from build123d import *

# Parameters (mm, degrees)
F0_W     = 15.8
F0_H     = 31.8
F0_R     = 2.4
F1_DEPTH = 9.6
F2_DEPTH = 11.4
F3_T     = -1.2
F5_W     = 0.6
F5_H     = 0.6
F6_DEPTH = 8.4
F4_R     = 3.25
F4_R_2   = 2.4
F7_DEPTH = 8.4
F8_START = 1.5
F8_DEPTH = 6.9


with BuildPart() as f1:
    # F0 (on Top) → F1 (new body)
    with BuildSketch(Plane.XY):
        Rectangle(F0_W, F0_H)
        with Locations((-4, -12)):
            Circle(F0_R, mode=Mode.SUBTRACT)
        with Locations((-4, -4)):
            Circle(F0_R, mode=Mode.SUBTRACT)
        with Locations((4, -12)):
            Circle(F0_R, mode=Mode.SUBTRACT)
        with Locations((4, -4)):
            Circle(F0_R, mode=Mode.SUBTRACT)
        with Locations((-4, 4)):
            Circle(F0_R, mode=Mode.SUBTRACT)
        with Locations((-4, 12)):
            Circle(F0_R, mode=Mode.SUBTRACT)
        with Locations((4, 4)):
            Circle(F0_R, mode=Mode.SUBTRACT)
        with Locations((4, 12)):
            Circle(F0_R, mode=Mode.SUBTRACT)
        with Locations((4, 4)):
            Circle(F0_R)
        with Locations((4, 12)):
            Circle(F0_R)
        with Locations((4, -4)):
            Circle(F0_R)
        with Locations((4, -12)):
            Circle(F0_R)
        with Locations((-4, -12)):
            Circle(F0_R)
        with Locations((-4, -4)):
            Circle(F0_R)
        with Locations((-4, 4)):
            Circle(F0_R)
        with Locations((-4, 12)):
            Circle(F0_R)
    extrude(amount=F1_DEPTH)

    # F0 (on Top) → F2 (join)
    with BuildSketch(Plane.XY):
        with Locations((-4, 12)):
            Circle(F0_R)
        with Locations((4, 12)):
            Circle(F0_R)
        with Locations((4, 4)):
            Circle(F0_R)
        with Locations((4, -4)):
            Circle(F0_R)
        with Locations((-4, -4)):
            Circle(F0_R)
        with Locations((-4, 4)):
            Circle(F0_R)
        with Locations((-4, -12)):
            Circle(F0_R)
        with Locations((4, -12)):
            Circle(F0_R)
    extrude(amount=F2_DEPTH)

    # F3
    f3_openings = [f1.faces().sort_by_distance(p)[0] for p in [
        (0, 0, 0),
    ]]
    offset(amount=F3_T, openings=f3_openings, kind=Kind.INTERSECTION)

    # F5 (on Top) → F6 (join, through all)
    with BuildSketch(Plane.XY):
        with Locations((-4, -14.7)):
            Rectangle(F5_W, F5_H)
        with Locations((4, -14.7)):
            Rectangle(F5_W, F5_H)
        with Locations((6.7, -12)):
            Rectangle(F5_W, F5_H)
        with Locations((-6.7, -12)):
            Rectangle(F5_W, F5_H)
        with Locations((-6.7, -4)):
            Rectangle(F5_W, F5_H)
        with Locations((6.7, -4)):
            Rectangle(F5_W, F5_H)
        with Locations((-6.7, 4)):
            Rectangle(F5_W, F5_H)
        with Locations((6.7, 4)):
            Rectangle(F5_W, F5_H)
        with Locations((6.7, 12)):
            Rectangle(F5_W, F5_H)
        with Locations((-6.7, 12)):
            Rectangle(F5_W, F5_H)
        with Locations((-4, 14.7)):
            Rectangle(F5_W, F5_H)
        with Locations((4, 14.7)):
            Rectangle(F5_W, F5_H)
    extrude(amount=F6_DEPTH)

    # F4 (on Top) → F7 (join, through all)
    with BuildSketch(Plane.XY):
        with Locations((0, -8)):
            Circle(F4_R)
        with Locations((0, -8)):
            Circle(F4_R_2, mode=Mode.SUBTRACT)
        with BuildLine():
            ThreePointArc((3.2361242251, -0.3), (3.246529203, -0.1501603619), (3.25, 0))
            ThreePointArc((3.25, 0), (3.246529203, 0.1501603619), (3.2361242251, 0.3))
            ThreePointArc((3.2361242251, 0.3), (0, 3.25), (-3.2361242251, 0.3))
            ThreePointArc((-3.2361242251, 0.3), (-3.25, 0), (-3.2361242251, -0.3))
            ThreePointArc((-3.2361242251, -0.3), (0, -3.25), (3.2361242251, -0.3))
        make_face()
        Circle(F4_R_2, mode=Mode.SUBTRACT)
        with Locations((0, 8)):
            Circle(F4_R)
        with Locations((0, 8)):
            Circle(F4_R_2, mode=Mode.SUBTRACT)
    extrude(amount=F7_DEPTH)

    # F4 (on Top) → F8 (join)
    with BuildSketch(Plane.XY.offset(F8_START)):
        with BuildLine():
            ThreePointArc((-3.2361242251, -0.3), (-3.25, 0), (-3.2361242251, 0.3))
            Line((-3.2361242251, 0.3), (-6.7, 0.3))
            Line((-6.7, 0.3), (-6.7, -0.3))
            Line((-6.7, -0.3), (-3.2361242251, -0.3))
        make_face()
        with BuildLine():
            ThreePointArc((3.2361242251, 0.3), (3.246529203, 0.1501603619), (3.25, 0))
            ThreePointArc((3.25, 0), (3.246529203, -0.1501603619), (3.2361242251, -0.3))
            Line((3.2361242251, -0.3), (6.7, -0.3))
            Line((6.7, -0.3), (6.7, 0.3))
            Line((6.7, 0.3), (3.2361242251, 0.3))
        make_face()
    extrude(amount=F8_DEPTH)


solid = f1.part
CAD build for the part. Positions are in the model's coordinates, mm. A direction names the side the tool comes from. Round coordinates to 2 decimals unless told otherwise and drop trailing zeros. Loops run counter-clockwise (first coordinate to the right, second up) from the corner with the lowest first, then second, coordinate; pieces in that order, holes last.
(1) Two-plate mould, pull along Y, no slides. Class faces 4 (the flat face through (4, -12, 11.4)), 5 (the flat face through (-4, 12, 10.2)): +Y half, -Y half, draft (parallel to the pull), parting line (faces both ways), or undercut.
(2) Drop flat-ended pins along their axis: pin 1 (4 mm diameter, centred on x = 0.5, y = 0, fed in from +Z); pin 2 (1.9 mm diameter, centred on x = -4, y = 12, fed in from -Z). Give the stop position or say it passes through.
(3) Cut at B-B (y = -4). Give the cut face in (x, z).
(4) Cut at A-A (z = 3.75). State how many separate pieces and enclosed holes the cut face has, plus the area to 3 significant figures.
(5) Which spindle directions (+Z, -Z, +X, -X, +Y, -Y) get a long thin tool onto all of the face, cutting with end or side? Do faces 1 (the flat face through (-7.9, 0, 5)), 2 (the cylindrical face through (1.29, 10.024, 4.141)), 3 (the cylindrical face through (6.29, -3.28, 10.49)). Say none if no direction does.
(6) Wall check: line 1 along Y through (x, z) = (4, 9.35); line 2 along Y through (x, z) = (4.25, 7.5); line 3 along X through (y, z) = (-12, 9.5). Give the ranges that are in metal, low to high.
Findings below:
1. face 4: draft
1. face 5: undercut
2. pin 1: stops at z = 9.6
2. pin 2: stops at z = 10.2
3. outline: (-7.9, 0) - (-6.4, 0) - (-6.4, 8.4) - (-5.2, 8.4) - (-5.2, 10.2) - (-2.8, 10.2) - (-2.8, 8.4) - (2.8, 8.4) - (2.8, 10.2) - (5.2, 10.2) - (5.2, 8.4) - (6.4, 8.4) - (6.4, 0) - (7.9, 0) - (7.9, 9.6) - (6.4, 9.6) - (6.4, 11.4) - (1.6, 11.4) - (1.6, 9.6) - (-1.6, 9.6) - (-1.6, 11.4) - (-6.4, 11.4) - (-6.4, 9.6) - (-7.9, 9.6) - close
4. separate pieces: 3
4. enclosed holes: 5
4. area: 160 mm2
5. face 1: +Z, -Z, -X, +Y, -Y
5. face 2: -Z
5. face 3: +Z
6. line 1: y = -15.9 to -13.2, -10.8 to -5.2, -2.8 to 2.8, 5.2 to 10.8, 13.2 to 15.9
6. line 2: y = -15.9 to -14.4, -0.3 to 0.3, 14.4 to 15.9
6. line 3: x = -7.9 to -5.2, -2.8 to 2.8, 5.2 to 7.9
